Verification items for the finished model (mm, model axes). A direction names the side the tool comes from. Coordinates: 2 decimals unless noted, no trailing zeros. Use one line per item in the form item = value. Start each with the question number.
(1) Gauge pin test, flat ends, axial feed: pin 1 Ø3 at (y, z) = (6.5, -3.5) entering from -X; pin 2 Ø1.2 at (y, z) = (6, 0) entering from +X; pin 3 Ø5 at (x, y) = (-3, -15.5) entering from +Z. Record the tip position at first contact, or that the pin passes through.
(2) Material ranges on line 1 (X direction, y = 12, z = 0); line 2 (X direction, y = -11, z = -3.5); line 3 (X direction, y = -17.5, z = 0.75), recorded low to high. Write a range as [from, to].
(3) Mould release check, pull along Y, two halves, no side actions. Record for faces 1 (the flat face through (-3, 15.5, -2)), 2 (the flat face through (-3.5, 4, 0)), 3 (the cylindrical face through (3.5, -9.3, 4.5)), 4 (the conical face through (1.931, -16.181, -1.004)): released by +Y, released by -Y, zero draft, split by the parting line, or undercut.
(4) Tool access check on faces 5 (the flat face through (3.5, 4, 0)), 6 (the cylindrical face through (-1.947, 10.817, -2.539)). Record the directions out of +Z, -Z, +X, -X, +Y, -Y that give a thin tool (end or side, any length) a straight path to the whole face; none if there is none.
from build123d import *

# Parameters (mm, degrees)
SKETCH2_R               = 3.2
CUT_EXTRUDE1_DEPTH      = 9.5
CUT_EXTRUDE2_DEPTH      = 9.5
CUT_EXTRUDE2_DEPTH_BACK = 9.5
SKETCH3_W               = 4
SKETCH3_H               = 9


with BuildPart() as part:
    # Sketch1 → Revolve1 (revolve)
    with BuildSketch(Plane.XY, mode=Mode.PRIVATE) as revolve1_sk:
        Polygon((0, -7.607142857), (0, 15.5), (-4, 15.5), (-4, -7), (-5.7, -8.5), (-5.7, -10), (0, -20), align=None)
    revolve(revolve1_sk.sketch.rotate(Axis((0, -7.607142857, 0), (0, 1, 0)), 270), axis=Axis((0, -7.607142857, 0), (0, 1, 0)))

    # Sketch2 → Cut-Extrude1 (cut)
    with BuildSketch(Plane(origin=(0, 15.5, 0), x_dir=(1, 0, 0), z_dir=(0, 1, 0))):
        with Locations(Location((0, 0, 0), (0, 0, 270))):
            Circle(SKETCH2_R)
    extrude(amount=-CUT_EXTRUDE1_DEPTH, mode=Mode.SUBTRACT)

    # Sketch3 → Cut-Extrude2 (cut, two sides: drawn at the far end of the back side and taken through both)
    with BuildSketch(Plane.XY.offset(-CUT_EXTRUDE2_DEPTH_BACK)):
        with Locations((-5.5, 4)):
            Rectangle(SKETCH3_W, SKETCH3_H)
        with Locations((5.5, 4)):
            Rectangle(SKETCH3_W, SKETCH3_H)
    extrude(amount=CUT_EXTRUDE2_DEPTH + CUT_EXTRUDE2_DEPTH_BACK, mode=Mode.SUBTRACT)


solid = part.part
Answers below:
q1.pin_1 = -3.46
q1.pin_2 = 3.5
q1.pin_3 = 3.39
q2.line_1 = [-4, -3.2], [3.2, 4]
q2.line_2 = [-3.75, 3.75]
q2.line_3 = [-1.21, 1.21]
q3.face_1 = released by +Y
q3.face_2 = undercut
q3.face_3 = zero draft
q3.face_4 = released by -Y
q4.face_5 = +Z, -Z, +X
q4.face_6 = +Y
